Could you check a few things on this model? Use its own coordinates, in mm. A direction names the side the tool comes from. Coordinates: 2 decimals unless noted, no trailing zeros. Order: outer loops, then holes, each group sorted by start corner. A loop starts at its lowest first (then second) coordinate and runs counter-clockwise, first axis right, second up. Notation, with made-up numbers: (-38.75, 34.25) -> (-32.75, 34.25) arc R6 ccw to (-32.75, 40.25) -> close; hole circle Ø2 at (15.25, -11.75). An arc over 180 degrees is marked (long way). Use a Markdown table: item, result. Add a question column.
1) Will these pins go through, and if not, where does the flat tip stop? pin 1 Ø10 at (x, y) = (6, 8.5) entering from +Z; pin 2 Ø8 at (y, z) = (18.5, -27.5) entering from +X; pin 3 Ø5 at (x, y) = (51, 12) entering from -Z; pin 4 Ø10 at (x, z) = (-30, -60) entering from +Y.
2) Thinking about a two-plate mould opening in Z: for faces 1 (the flat face through (-50, 13, -5.08)), 2 (the flat face through (48, 13, 0)), 3 (the flat face through (0, 12.7, -60)), which applies, +Z half, -Z half, draft (parallel to the pull), parting line (faces both ways), or undercut?
3) If we section it at A-A (z = -34): Write out the boundary of the cut face in (x, y).
4) Which directions (+Z, -Z, +X, -X, +Y, -Y) give clear straight access to the entire face, cutting with the end or side of a thin tool? Please do faces 4 (the flat face through (-24.77, 6.44, -54.26)), 5 (the flat face through (55.161, 13, -3)), 6 (the flat face through (-39.912, 13, -1)).
5) If I drill on L1, parallel to Z at x = 0.5, y = 6; L2, parallel to Z at x = -15.5, y = 9.5; L3, parallel to X at y = 1, z = -14.5, over which ranges is the centre line in solid material (lowest first)? Write a range as [from, to].
6) If we section it at C-C (x = 0): Write out the boundary of the cut face in (y, z), plus the area to 3 significant figures.
7) If we section it at B-B (y = 6.25): Write out the boundary of the cut face in (x, z), plus the area to 3 significant figures.
8) If we section it at D-D (z = -52.5): Write out the boundary of the cut face in (x, y).
```python
from build123d import *

# Parameters (mm, degrees)
SKETCH1_R               = 45.0723
SKETCH1_R_2             = 39.9923
BOSS_EXTRUDE1_DEPTH     = 25.4
BOSS_EXTRUDE2_DEPTH     = 12.7
BOSS_EXTRUDE3_DEPTH     = 12.7
SKETCH4_W               = 90.1446
SKETCH4_H               = 25.4
CUT_EXTRUDE1_DEPTH      = 46.0723
CUT_EXTRUDE1_DEPTH_BACK = 2.54
BOSS_EXTRUDE4_DEPTH     = 2.54


with BuildPart() as part:
    # Sketch1 → Boss-Extrude1 (new body)
    with BuildSketch(Plane(origin=(0, 0, 0), x_dir=(1, 0, 0), z_dir=(0, 1, 0))):
        Circle(SKETCH1_R)
        Circle(SKETCH1_R_2, mode=Mode.SUBTRACT)
    extrude(amount=BOSS_EXTRUDE1_DEPTH)

    # Sketch2 → Boss-Extrude2 (add, symmetric)
    with BuildSketch(Plane(origin=(0, 12.7, 0), x_dir=(1, 0, 0), z_dir=(0, 1, 0))):
        Polygon((45.0723, 0), (19.05, 80.085348852), (-19.05, 80.085348852), (-45.0723, 0), (-42.65662525, -0.784930252), (-17.204603736, 77.545348852), (17.204603736, 77.545348852), (42.65662525, -0.784930252), align=None)
    extrude(amount=BOSS_EXTRUDE2_DEPTH, both=True)

    # Sketch3 → Boss-Extrude3 (add)
    with BuildSketch(Plane(origin=(0, 25.4, 0), x_dir=(1, 0, 0), z_dir=(0, 1, 0))):
        with BuildLine():
            Line((-17.204603736, 77.545348852), (17.204603736, 77.545348852))
            Line((17.204603736, 77.545348852), (32.130834652, 31.60888628))
            ThreePointArc((32.130834652, 31.60888628), (0, 45.0723), (-32.130834652, 31.60888628))
            Line((-32.130834652, 31.60888628), (-17.204603736, 77.545348852))
        make_face()
    extrude(amount=-BOSS_EXTRUDE3_DEPTH)

    # Sketch4 → Cut-Extrude1 (cut, two sides)
    with BuildSketch(Plane.XY) as cut_extrude1_sk:
        with Locations((0, 12.7)):
            Rectangle(SKETCH4_W, SKETCH4_H)
    extrude(amount=CUT_EXTRUDE1_DEPTH, mode=Mode.SUBTRACT)
    extrude(cut_extrude1_sk.sketch, amount=-CUT_EXTRUDE1_DEPTH_BACK, mode=Mode.SUBTRACT)

    # Sketch5 → Boss-Extrude4 (add, symmetric)
    with BuildSketch(Plane.XY.offset(-2.54)):
        Polygon((-45.000673632, 25.4), (-39.911557966, 25.4), (-39.911557966, 0), (-45.086454025, 0), (-55.160673632, 0), (-55.160673632, 25.4), align=None)
        Polygon((55.160673632, 25.4), (55.160673632, 0), (45.086454025, 0), (39.911557966, 0), (39.911557966, 25.4), (45.000673632, 25.4), align=None)
    extrude(amount=BOSS_EXTRUDE4_DEPTH, both=True)


solid = part.part
```
Answer sheet:
| question | item | result |
|---|---|---|
| 1 | pin 1 | z = -38.45 |
| 1 | pin 2 | x = 38.46 |
| 1 | pin 3 | z = -5.08 |
| 1 | pin 4 | y = 25.4 |
| 2 | face 1 | -Z half |
| 2 | face 2 | +Z half |
| 2 | face 3 | undercut |
| 3 | outline | (-34.02, 0) -> (-31.35, 0) -> (-31.35, 12.7) -> (-29.59, 12.7) -> (-29.59, 0) -> (-21.06, 0) -> (-21.06, 25.4) -> (-34.02, 25.4) -> close; (21.06, 0) -> (29.59, 0) -> (29.59, 12.7) -> (31.35, 12.7) -> (31.35, 0) -> (34.02, 0) -> (34.02, 25.4) -> (21.06, 25.4) -> close |
| 4 | face 4 | -Y |
| 4 | face 5 | +Z, -Z, +X, +Y, -Y |
| 4 | face 6 | +Z, +Y, -Y |
| 5 | L1 | [-80.09, -77.55], [-45.07, -39.99] |
| 5 | L2 | [-80.09, -77.55], [-42.32, -36.87] |
| 5 | L3 | [-42.68, -37.27], [37.27, 42.68] |
| 6 | outline | (0, -80.09) -> (25.4, -80.09) -> (25.4, -39.99) -> (0, -39.99) -> (0, -45.07) -> (12.7, -45.07) -> (12.7, -77.55) -> (0, -77.55) -> close |
| 6 | area | 606 mm2 |
| 7 | outline | (-55.16, -5.08) -> (-44.79, -5.08) arc R45.07 ccw to (-36.46, -26.49) -> (-19.05, -80.09) -> (19.05, -80.09) -> (36.46, -26.49) arc R45.07 ccw to (44.79, -5.08) -> (55.16, -5.08) -> (55.16, 0) -> (39.91, 0) -> (39.91, -2.54) arc R39.99 cw to (-39.91, -2.54) -> (-39.91, 0) -> (-55.16, 0) -> close; hole (-32.13, -31.61) -> (-17.2, -77.55) -> (17.2, -77.55) -> (32.13, -31.61) arc R45.07 cw to start |
| 7 | area | 1,140 mm2 |
| 8 | outline | (-28.01, 0) -> (-25.34, 0) -> (-25.34, 12.7) -> (25.34, 12.7) -> (25.34, 0) -> (28.01, 0) -> (28.01, 25.4) -> (-28.01, 25.4) -> close |
